Autodesk Inventor part; units mm, degrees
ref_plane "YZ Plane" through (0, 0, 0) normal (1, 0, 0) x (0, 1, 0)
ref_plane "XZ Plane" through (0, 0, 0) normal (0, 1, 0) x (-1, 0, 0)
ref_plane "XY Plane" through (0, 0, 0) normal (0, 0, 1) x (1, 0, 0)
sketch "Sketch1" plane through (0, 0, 0) normal (0, 1, 0) x (-1, 0, 0)
  arc A0 (-1.4, -51.2845) -> (-1.4, -48.7155) centre (0, -50) ccw
  line L0 (-1.4, -48.7155) -> (-1.4, -51.2845)
  line L1 (-2.1842, 109.6159) -> (-1.9664, 109.7389)
  arc A1 (1.9664, 109.7389) -> (-1.9664, 109.7389) centre (0, 106.2556) ccw
  line L2 (1.9664, 109.7389) -> (2.1842, 109.6159)
  arc A2 (3.5277, 108.3788) -> (2.1842, 109.6159) centre (0.2179, 106.1326) ccw
  line L3 (3.5277, 108.3788) -> (8.2122, 101.4762)
  arc A3 (8.9023, 99.2105) -> (8.2122, 101.4762) centre (4.9024, 99.23) ccw
  line L4 (8.9023, 99.2105) -> (8.5178, 20.4265)
  arc A4 (5.6167, -33.4003) -> (8.5178, -29.5737) centre (4.5178, -29.5542) ccw
  line L5 (5.6167, -33.4003) -> (1.0989, -34.6911)
  arc A5 (-1.0989, -34.6911) -> (1.0989, -34.6911) centre (0, -30.845) ccw
  line L6 (-1.0989, -34.6911) -> (-5.6167, -33.4003)
  arc A6 (-8.5178, -29.5737) -> (-5.6167, -33.4003) centre (-4.5178, -29.5542) ccw
  line L7 (-8.5178, 20.4265) -> (-8.9023, 99.2105)
  arc A7 (-8.2122, 101.4762) -> (-8.9023, 99.2105) centre (-4.9024, 99.23) ccw
  line L8 (-8.2122, 101.4762) -> (-3.5277, 108.3788)
  arc A8 (-2.1842, 109.6159) -> (-3.5277, 108.3788) centre (-0.2179, 106.1326) ccw
  line L9 (-3.9333, 127.6797) -> (-4.4928, 131.0366)
  arc A9 (-4.4182, 132.354) -> (-4.4928, 131.0366) centre (-1.5336, 131.5298) ccw
  line L10 (-4.4182, 132.354) -> (-4.2433, 132.9662)
  arc A10 (-1.3587, 135.1421) -> (-4.2433, 132.9662) centre (-1.3587, 132.1421) ccw
  line L11 (-1.3587, 135.1421) -> (1.3587, 135.1421)
  arc A11 (4.2433, 132.9662) -> (1.3587, 135.1421) centre (1.3587, 132.1421) ccw
  line L12 (4.2433, 132.9662) -> (4.4182, 132.354)
  arc A12 (4.4928, 131.0366) -> (4.4182, 132.354) centre (1.5336, 131.5298) ccw
  line L13 (4.4928, 131.0366) -> (3.9333, 127.6797)
  arc A13 (1.7983, 125.2884) -> (3.9333, 127.6797) centre (0.9742, 128.1729) ccw
  line L14 (1.7983, 125.2884) -> (0.8242, 125.01)
  arc A14 (-0.8242, 125.01) -> (0.8242, 125.01) centre (0, 127.8946) ccw
  line L15 (-0.8242, 125.01) -> (-1.7983, 125.2884)
  arc A15 (-3.9333, 127.6797) -> (-1.7983, 125.2884) centre (-0.9742, 128.1729) ccw
  arc A16 (-12.5, 127.1805) -> (-11.6588, 124.7265) centre (-8.5, 127.1805) ccw
  line L16 (-11.6588, 124.7265) -> (-8.4827, 120.6384)
  arc A17 (-7.6415, 118.1843) -> (-8.4827, 120.6384) centre (-11.6415, 118.1843) ccw
  line L17 (-7.6415, 118.1843) -> (-7.6415, 112.7784)
  arc A18 (-8.147, 110.832) -> (-7.6415, 112.7784) centre (-11.6415, 112.7784) ccw
  line L18 (-8.147, 110.832) -> (-11.9945, 103.9244)
  arc A19 (-11.9945, 103.9244) -> (-12.5, 101.978) centre (-8.5, 101.978) ccw
  line L19 (-12.5, 101.978) -> (-12.5, 0)
  arc A20 (-12.5, -50) -> (12.5, -50) centre (0, -50) ccw
  line L20 (12.5, 0) -> (12.5, 101.978)
  arc A21 (12.5, 101.978) -> (11.9945, 103.9244) centre (8.5, 101.978) ccw
  line L21 (11.9945, 103.9244) -> (8.147, 110.832)
  arc A22 (7.6415, 112.7784) -> (8.147, 110.832) centre (11.6415, 112.7784) ccw
  line L22 (7.6415, 112.7784) -> (7.6415, 118.1843)
  arc A23 (8.4827, 120.6384) -> (7.6415, 118.1843) centre (11.6415, 118.1843) ccw
  line L23 (8.4827, 120.6384) -> (11.6588, 124.7265)
  arc A24 (11.6588, 124.7265) -> (12.5, 127.1805) centre (8.5, 127.1805) ccw
  line L24 (12.5, 127.1805) -> (12.5, 150)
  arc A25 (12.5, 150) -> (-12.5, 150) centre (0, 150) ccw
  line L25 (-12.5, 150) -> (-12.5, 127.1805)
  circle A26 centre (8.5, -50) radius 1.5
  circle A27 centre (-8.5, -50) radius 1.5
  circle A28 centre (0, 150) radius 4.5
  circle A29 centre (-8.5, 130) radius 1.6
  circle A30 centre (8.5, 130) radius 1.6
  circle A31 centre (-7.4, 150) radius 1.5
  circle A32 centre (7.4, 150) radius 1.5
  line L26 (0, 150) -> (0, -50)
  line L27 (0, -50) -> (0, -30.845)
  line L28 (12.5, 0) -> (12.5, -50)
  line L29 (-12.5, 0) -> (-12.5, -50)
  line L30 (-8.5178, 20.4265) -> (-8.5178, -29.5737)
  line L31 (8.5178, 20.4265) -> (8.5178, -29.5737)
  line L32 (7.4, 102.6729) -> (7.4, -32.3278)
  line L33 (-7.4, 102.6729) -> (-7.4, -32.3278)
  point P0 (0, 0)
  dimension "d0" = 200
  dimension "d1" = 19.155
extrude "Extrusion1" add sketch "Sketch1" along normal blind 5 contours A6 L30 L7 A7 L8 L33 | L32 L3 A3 L4 L31 A4 | L25 A25 L24 A24 L23 A23 L22 A22 L21 A21 L20 L28 A20 L29 L19 A19 L18 A18 L17 A17 L16 A16
fillet "Fillet1" radius 2.5 4 edges at (7.4, 2.5, 102.6729) (-7.4, 2.5, 102.6729) (7.4, 2.5, -32.3278) (-7.4, 2.5, -32.3278)
properties material "Polycarbonate, Clear"
The model under review builds one solid part; all positions refer to its coordinate system, in mm. A direction names the side the tool comes from. Give positions to 0.01 mm unless a question says otherwise; leave off trailing zeros. Write each loop counter-clockwise with the first axis right and the second up, starting at its lowest first coordinate (ties: lowest second). Pieces come first, ordered by that corner, then holes.
(1) For P1, Ø2.5, axis at y = 3, z = 116, coming from the +X side; P2, Ø1, axis at x = 8.5, y = 3, coming from the +Z side; P3, Ø7, axis at x = 0, z = 150, coming from the +Y side; P4, Ø2, axis at x = 8.5, y = 2.5, coming from the -Z side, all flat-tipped, find the tip position at first contact; note any pin that passes through.
(2) To check wall thickness, follow L1, parallel to Z at x = 0, y = 2.8 (3 decimals); L2, parallel to X at y = 3.35, z = 12.5; L3, parallel to Z at x = -3.25, y = 3.9. State the ranges of each line that lie inside material, in increasing order.
(3) The part is to be moulded in two halves that separate along X. For faces 4 (the flat face through (-10.049, 2.465, 122.654)), 5 (the flat face through (-3.374, 2.465, -34.041)), 6 (the cylindrical face through (0.275, 2.465, 162.497)), say which applies: released by +X, released by -X, zero draft, split by the parting line, or undercut.
(4) Tool access review of faces 1 (the flat face through (7.642, 2, 116)), 2 (the flat face through (-10.098, 2.465, 107.33)), 3 (the flat face through (7.4, 2, 36)): name each direction out of +Z, -Z, +X, -X, +Y, -Y from which nothing blocks a thin tool from reaching the whole face with its end or side.
(5) Consider section A-A, the plane z = 88. Give the boundary of the cut face in (x, y), and give its area (3 significant figures).
(6) Consider section B-B, the plane y = 1.9. Give the number of separate pieces and of enclosed holes in the cut face, and give its area (3 significant figures).
Returned:
1. P1: stops at x = 7.64
1. P2: stops at z = 159.6
1. P3: passes through
1. P4: stops at z = -60
2. L1: z = -62.5 to -51.9, -48.1 to -34.845, 110.256 to 124.895, 135.142 to 145.5, 154.5 to 162.5
2. L2: x = -12.5 to -7.4, 7.4 to 12.5
2. L3: z = -62.07 to -34.08, 108.74 to 126.22, 134.47 to 146.89, 153.11 to 162.07
3. face 4: released by -X
3. face 5: undercut
3. face 6: split by the parting line
4. face 1: +X, +Y, -Y
4. face 2: -X, +Y, -Y
4. face 3: +Y, -Y
5. outline: (-12.5, 0) - (-7.4, 0) - (-7.4, 5) - (-12.5, 5) - close; (7.4, 0) - (12.5, 0) - (12.5, 5) - (7.4, 5) - close
5. area: 51.0 mm2
6. separate pieces: 1
6. enclosed holes: 10
6. area: 3,050 mm2
